Design review of the part built by this model. Coordinates are the model's own, in mm. Face numbers are marked on the shaded views. A direction names the side the tool comes from. Round coordinates to 2 decimals unless told otherwise and drop trailing zeros. Order: outer loops, then holes, each group sorted by start corner. A loop starts at its lowest first (then second) coordinate and runs counter-clockwise, first axis right, second up. Notation, with made-up numbers: (82.5, 13) - (135.5, 13) arc R30 ccw to (135.5, 37) - close; hole circle Ø11 at (-9.5, -10). An arc over 180 degrees is marked (long way). Write item = value, one per line.
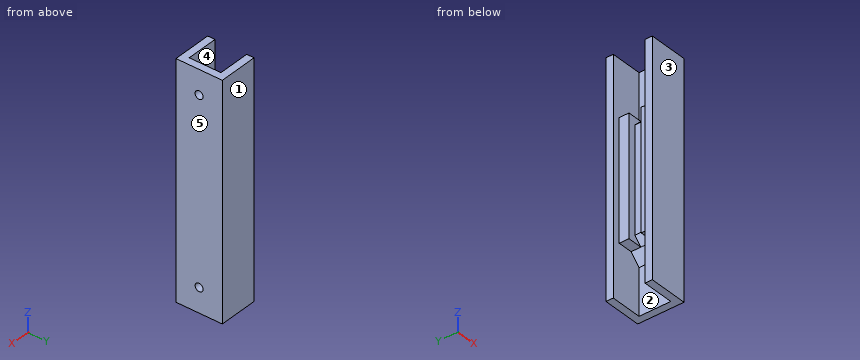
from build123d import *

# Parameters (mm, degrees)
SKETCH_1_W          = 19
SKETCH_1_H          = 19
SKETCH_1_W_2        = 13
SKETCH_1_H_2        = 13
EXTRUDE_1_DEPTH     = 95
SKETCH_2_R          = 1.65
CUT_EXTRUDE_1_DEPTH = 30
SKETCH_3_W          = 116.915177823
SKETCH_3_H          = 46.219516436
CUT_EXTRUDE_2_DEPTH = 3
SKETCH_4_W          = 5
SKETCH_4_H          = 13
EXTRUDE_1_2_DEPTH   = 10
SKETCH_5_W          = 39
SKETCH_5_H          = 5
EXTRUDE_2_DEPTH     = 10
SKETCH_6_W          = 49
SKETCH_6_H          = 13
EXTRUDE_3_DEPTH     = 10
SKETCH_8_W          = 49
SKETCH_8_H          = 5
CUT_EXTRUDE_3_DEPTH = 3
CHAMFER_1_SIZE      = 3
CHAMFER_2_SIZE      = 4


with BuildPart() as part:
    # 草图1 → Extrude 1 (new body)
    with BuildSketch(Plane.XY):
        with Locations((6.5, 6.5)):
            Rectangle(SKETCH_1_W, SKETCH_1_H)
        with Locations((6.5, 6.5)):
            Rectangle(SKETCH_1_W_2, SKETCH_1_H_2, mode=Mode.SUBTRACT)
    extrude(amount=EXTRUDE_1_DEPTH)

    # 草图2 → 切除-拉伸1 (cut)
    with BuildSketch(Plane.ZY.offset(3)):
        with Locations((10, 6.5)):
            Circle(SKETCH_2_R)
        with Locations((85, 6.5)):
            Circle(SKETCH_2_R)
    extrude(amount=-CUT_EXTRUDE_1_DEPTH, mode=Mode.SUBTRACT)

    # 草图3 → 切除-拉伸2 (cut)
    with BuildSketch(Plane.ZY.offset(3)):
        with Locations((53.162237228, 0.202739406)):
            Rectangle(SKETCH_3_W, SKETCH_3_H)
    extrude(amount=-CUT_EXTRUDE_2_DEPTH, mode=Mode.SUBTRACT)

    # 草图4 → Extrude 1 2 (add)
    with BuildSketch(Plane.ZY.offset(-13)):
        with Locations((25.5, 6.5)):
            Rectangle(SKETCH_4_W, SKETCH_4_H)
        with Locations((69.5, 6.5)):
            Rectangle(SKETCH_4_W, SKETCH_4_H)
    extrude(amount=EXTRUDE_1_2_DEPTH)

    # 草图5 → 凸台-拉伸2 (add)
    with BuildSketch(Plane.ZY.offset(-13)):
        with Locations((47.5, 6.5)):
            Rectangle(SKETCH_5_W, SKETCH_5_H)
    extrude(amount=EXTRUDE_2_DEPTH)

    # 草图6 → 凸台-拉伸3 (add)
    with BuildSketch(Plane.ZY.offset(-13)):
        with Locations((47.5, 6.5)):
            Rectangle(SKETCH_6_W, SKETCH_6_H)
    extrude(amount=EXTRUDE_3_DEPTH)

    # 草图8 → 切除-拉伸3 (cut)
    with BuildSketch(Plane.ZY.offset(-3)):
        with Locations((47.5, 6.5)):
            Rectangle(SKETCH_8_W, SKETCH_8_H)
    extrude(amount=-CUT_EXTRUDE_3_DEPTH, mode=Mode.SUBTRACT)

    # 倒角1
    chamfer_1_edges = [part.edges().sort_by_distance(p)[0] for p in [
        (6, 6.5, 23),
        (6, 6.5, 72),
    ]]
    chamfer(chamfer_1_edges, length=CHAMFER_1_SIZE)

    # 倒角2
    chamfer_2_edges = [part.edges().sort_by_distance(p)[0] for p in [
        (13, 6.5, 23),
        (13, 6.5, 72),
    ]]
    chamfer(chamfer_2_edges, length=CHAMFER_2_SIZE - 0.0001)  # a hair under: the kernel refuses the full size


solid = part.part
Item 1: The part is to be moulded in two halves that separate along Y. For the marked faces 1, 2 and 3, say which applies: +Y half, -Y half, draft (parallel to the pull), parting line (faces both ways), or undercut.
Data:
face_1 = +Y half
face_2 = undercut
face_3 = -Y half
Item 2: Take a section at A-A, the plane x = 1.75. State the section outline as (y, z) points, and give its area (3 significant figures).
Data:
outline = (-3, 0) - (0, 0) - (0, 95) - (-3, 95) - close; (13, 0) - (16, 0) - (16, 95) - (13, 95) - close
area = 570 mm2
Item 3: Take a section at C-C, the plane z = 85. State the section outline as (x, y) points, and give its area (3 significant figures).
Data:
outline = (0, -3) - (16, -3) - (16, 4.85) - (13, 4.85) - (13, 0) - (0, 0) - close; (0, 13) - (13, 13) - (13, 8.15) - (16, 8.15) - (16, 16) - (0, 16) - close
area = 125 mm2
Item 4: For the marked faces 4 and 5, list the 3-axis set-ups (+Z, -Z, +X, -X, +Y, -Y) from which the entire face can be reached by the end or side of a thin tool; tool diameter is ignored.
Data:
face_4 = -X
face_5 = +Z, -Z, +X, +Y, -Y
Item 5: Take a section at D-D, the plane y = 6.5. Count the separate pieces of the cut face and the enclosed holes in it, and give its area (3 significant figures).
Data:
separate_pieces = 3
enclosed_holes = 0
area = 615 mm2
Item 6: For line 1 along Y through (x, z) = (13.65, 85); line 2 along Y through (x, z) = (4.25, 47.5); line 3 along X through (y, z) = (1, 44), list the stretches that pass through material, from the lowest coordinate up. Write a range as [from, to].
Data:
line_1 = [-3, 4.85], [8.15, 16]
line_2 = [-3, 4], [9, 16]
line_3 = [3, 16]
Item 7: Take a section at B-B, the plane y = 10. State the section outline as (x, z) points.
Data:
outline = (3, 23) - (9, 23) - (13, 19) - (13, 0) - (16, 0) - (16, 95) - (13, 95) - (13, 76) - (9, 72) - (3, 72) - close
Item 8: Insertion check: P1, Ø2.5, axis at y = 6.5, z = 85, coming from the -X side; P2, Ø6.5, axis at x = 6.5, y = 5, coming from the -Z side; P3, Ø5.5, axis at y = 6.5, z = 10, coming from the -X side; P4, Ø3, axis at y = 2, z = 49.5, coming from the -X side. Each pin has a flat end and moves straight along its axis. Give the tip position at first contact, or say it passes through.
Data:
P1 = through
P2 = 22.25
P3 = 13
P4 = 3
